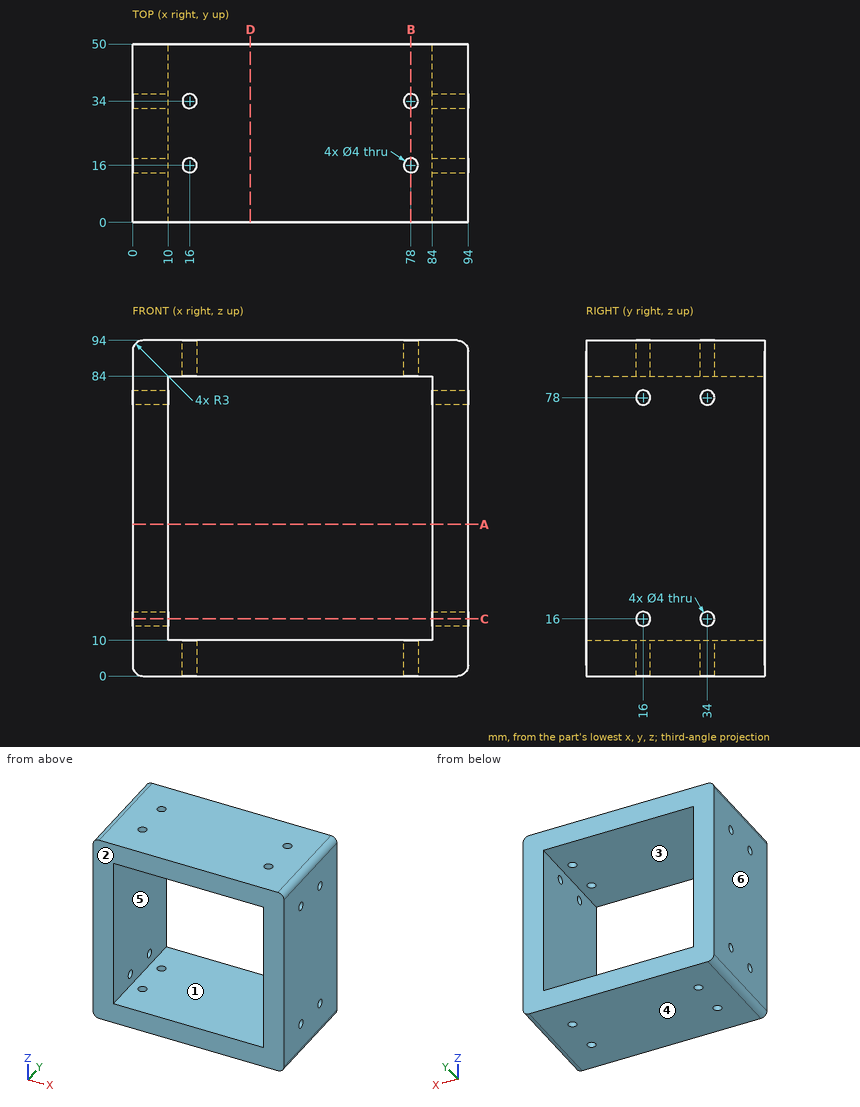
Here's the drawing with two shaded views (mm, measured from the low corner). I have some questions. A direction names the side the tool comes from. Round coordinates to 2 decimals unless told otherwise and drop trailing zeros. Order: outer loops, then holes, each group sorted by start corner. A loop starts at its lowest first (then second) coordinate and runs counter-clockwise, first axis right, second up. Notation, with made-up numbers: (80, -5.5) -> (136, -5.5) arc R20 ccw to (136, 24.5) -> close; hole circle Ø2 at (-18.75, 50.5). An arc over 180 degrees is marked (long way). Return JSON: item names as keys, results as strings.
Q1. If we section it at C-C on z = 16: List the corners of the cut face in (x, y) for me.
Filled sheet:
{"outline": "(0, 0) -> (10, 0) -> (10, 14) -> (0, 14) -> close; (0, 18) -> (10, 18) -> (10, 32) -> (0, 32) -> close; (0, 36) -> (10, 36) -> (10, 50) -> (0, 50) -> close; (84, 0) -> (94, 0) -> (94, 14) -> (84, 14) -> close; (84, 18) -> (94, 18) -> (94, 32) -> (84, 32) -> close; (84, 36) -> (94, 36) -> (94, 50) -> (84, 50) -> close"}
Q2. If we section it at D-D on x = 33: List the corners of the cut face in (y, z) for me, plus the area to 3 significant figures.
Filled sheet:
{"outline": "(0, 0) -> (50, 0) -> (50, 10) -> (0, 10) -> close; (0, 84) -> (50, 84) -> (50, 94) -> (0, 94) -> close", "area": "1,000 mm^2"}
Q3. If we mould it in two halves opening along X, with no side actions, what happens to the marked faces 3, 4, 5 and 6? For each: released by +X, released by -X, zero draft, split by the parting line, or undercut.
Filled sheet:
{"face 3": "undercut", "face 4": "zero draft", "face 5": "undercut", "face 6": "released by -X"}
Q4. If we section it at B-B on x = 78: List the corners of the cut face in (y, z) for me.
Filled sheet:
{"outline": "(0, 0) -> (14, 0) -> (14, 10) -> (0, 10) -> close; (0, 84) -> (14, 84) -> (14, 94) -> (0, 94) -> close; (18, 0) -> (32, 0) -> (32, 10) -> (18, 10) -> close; (18, 84) -> (32, 84) -> (32, 94) -> (18, 94) -> close; (36, 0) -> (50, 0) -> (50, 10) -> (36, 10) -> close; (36, 84) -> (50, 84) -> (50, 94) -> (36, 94) -> close"}
Q5. If we section it at A-A on z = 42.5: List the corners of the cut face in (x, y) for me.
Filled sheet:
{"outline": "(0, 0) -> (10, 0) -> (10, 50) -> (0, 50) -> close; (84, 0) -> (94, 0) -> (94, 50) -> (84, 50) -> close"}
Q6. Which directions (+Z, -Z, +X, -X, +Y, -Y) give clear straight access to the entire face, cutting with the end or side of a thin tool? Please do the marked faces 1 and 2.
Filled sheet:
{"face 1": "+Y, -Y", "face 2": "+Z, -Z, +X, -X, -Y"}
Q7. I need wall thicknesses on line 1 along Y through (x, z) = (78, 4.25); line 2 along Z through (x, y) = (61, 19). Which ranges of each line are inside material? Lowest first, please. Write a range as from..to.
Filled sheet:
{"line 1": "y = 0..14, 18..32, 36..50", "line 2": "z = 0..10, 84..94"}
